```python
from build123d import *

# Parameters (mm, degrees)
SKETCH2_W                           = 10
SKETCH2_H                           = 25
F_5_6_5_6_DIAMETER_HOLE1_AT_2_COUNT = 2
F_5_6_5_6_DIAMETER_HOLE1_AT_2_PITCH = 17.5
F_5_6_5_6_DIAMETER_HOLE1_AT_3_COUNT = 2
F_5_6_5_6_DIAMETER_HOLE1_AT_3_PITCH = 30.310889132
F_5_6_5_6_DIAMETER_HOLE1_AT_4_COUNT = 2
F_5_6_5_6_DIAMETER_HOLE1_AT_4_PITCH = 35
F_5_6_5_6_DIAMETER_HOLE1_AT_5_COUNT = 2
F_5_6_5_6_DIAMETER_HOLE1_AT_5_PITCH = 30.310889132
F_5_6_5_6_DIAMETER_HOLE1_AT_6_COUNT = 2
F_5_6_5_6_DIAMETER_HOLE1_AT_6_PITCH = 17.5
F_0_5MM_CHAMFER1_SIZE               = 0.5


with BuildPart() as part:
    # Sketch2 → Revolve1 (revolve)
    with BuildSketch(Plane.XY, mode=Mode.PRIVATE) as revolve1_sk:
        with Locations((17.5, 12.5)):
            Rectangle(SKETCH2_W, SKETCH2_H)
    revolve1 = revolve(revolve1_sk.sketch.rotate(Axis((0, 0, 0), (0, 1, 0)), 90), axis=Axis((0, 0, 0), (0, 1, 0)))

    # Sketch5 → Ø5.6 (5.6) Diameter Hole1 (revolve, cut)
    with BuildSketch(Plane(origin=(15.155444566, 25, 8.75), x_dir=(0, 0, 1), z_dir=(1, 0, 0))):
        Polygon((0, 0), (0, 9.682409733), (2.8, 8), (2.8, 0), align=None)
    f_5_6_5_6_diameter_hole1 = revolve(axis=Axis((15.155444566, 31.35, 8.75), (0, -1, 0)), mode=Mode.SUBTRACT)

    # Ø5.6 (5.6) Diameter Hole1 at 2: Ø5.6 (5.6) Diameter Hole1 ×2
    with Locations(*[Vector(-0.8660254037844417, 0, 0.49999999999999495) * (i * F_5_6_5_6_DIAMETER_HOLE1_AT_2_PITCH) for i in range(1, F_5_6_5_6_DIAMETER_HOLE1_AT_2_COUNT)]):
        add(f_5_6_5_6_diameter_hole1, mode=Mode.SUBTRACT)

    # Ø5.6 (5.6) Diameter Hole1 at 3: Ø5.6 (5.6) Diameter Hole1 ×2
    with Locations(*[(-i * F_5_6_5_6_DIAMETER_HOLE1_AT_3_PITCH, 0, 0) for i in range(1, F_5_6_5_6_DIAMETER_HOLE1_AT_3_COUNT)]):
        add(f_5_6_5_6_diameter_hole1, mode=Mode.SUBTRACT)

    # Ø5.6 (5.6) Diameter Hole1 at 4: Ø5.6 (5.6) Diameter Hole1 ×2
    with Locations(*[Vector(-0.8660254037844346, 0, -0.5000000000000072) * (i * F_5_6_5_6_DIAMETER_HOLE1_AT_4_PITCH) for i in range(1, F_5_6_5_6_DIAMETER_HOLE1_AT_4_COUNT)]):
        add(f_5_6_5_6_diameter_hole1, mode=Mode.SUBTRACT)

    # Ø5.6 (5.6) Diameter Hole1 at 5: Ø5.6 (5.6) Diameter Hole1 ×2
    with Locations(*[Vector(-0.49999999999999195, 0, -0.8660254037844433) * (i * F_5_6_5_6_DIAMETER_HOLE1_AT_5_PITCH) for i in range(1, F_5_6_5_6_DIAMETER_HOLE1_AT_5_COUNT)]):
        add(f_5_6_5_6_diameter_hole1, mode=Mode.SUBTRACT)

    # Ø5.6 (5.6) Diameter Hole1 at 6: Ø5.6 (5.6) Diameter Hole1 ×2
    with Locations(*[(0, 0, -i * F_5_6_5_6_DIAMETER_HOLE1_AT_6_PITCH) for i in range(1, F_5_6_5_6_DIAMETER_HOLE1_AT_6_COUNT)]):
        add(f_5_6_5_6_diameter_hole1, mode=Mode.SUBTRACT)

    # Mirror1: Revolve1, Ø5.6 (5.6) Diameter Hole1 across plane
    add(revolve1.mirror(Plane.ZX))
    add(f_5_6_5_6_diameter_hole1.mirror(Plane.ZX), mode=Mode.SUBTRACT)

    # Mirror1 copy 1 sketch → Mirror1 copy 1 (revolve, cut)
    with BuildSketch(Plane(origin=(0, -25, 17.5), x_dir=(0, 0, 1), z_dir=(1, 0, 0))):
        Polygon((0, 0), (0, -9.682409733), (2.8, -8), (2.8, 0), align=None)
    revolve(axis=Axis((0, -31.35, 17.5), (0, -1, 0)), mode=Mode.SUBTRACT)

    # Mirror1 copy 2 sketch → Mirror1 copy 2 (revolve, cut)
    with BuildSketch(Plane(origin=(-15.155444566, -25, 8.75), x_dir=(0, 0, 1), z_dir=(1, 0, 0))):
        Polygon((0, 0), (0, -9.682409733), (2.8, -8), (2.8, 0), align=None)
    revolve(axis=Axis((-15.155444566, -31.35, 8.75), (0, -1, 0)), mode=Mode.SUBTRACT)

    # Mirror1 copy 3 sketch → Mirror1 copy 3 (revolve, cut)
    with BuildSketch(Plane(origin=(-15.155444566, -25, -8.75), x_dir=(0, 0, 1), z_dir=(1, 0, 0))):
        Polygon((0, 0), (0, -9.682409733), (2.8, -8), (2.8, 0), align=None)
    revolve(axis=Axis((-15.155444566, -31.35, -8.75), (0, -1, 0)), mode=Mode.SUBTRACT)

    # Mirror1 copy 4 sketch → Mirror1 copy 4 (revolve, cut)
    with BuildSketch(Plane(origin=(0, -25, -17.5), x_dir=(0, 0, 1), z_dir=(1, 0, 0))):
        Polygon((0, 0), (0, -9.682409733), (2.8, -8), (2.8, 0), align=None)
    revolve(axis=Axis((0, -31.35, -17.5), (0, -1, 0)), mode=Mode.SUBTRACT)

    # Mirror1 copy 5 sketch → Mirror1 copy 5 (revolve, cut)
    with BuildSketch(Plane(origin=(15.155444566, -25, -8.75), x_dir=(0, 0, 1), z_dir=(1, 0, 0))):
        Polygon((0, 0), (0, -9.682409733), (2.8, -8), (2.8, 0), align=None)
    revolve(axis=Axis((15.155444566, -31.35, -8.75), (0, -1, 0)), mode=Mode.SUBTRACT)

    # 0,5mm Chamfer1
    f_0_5mm_chamfer1_edges = [part.edges().sort_by_distance(p)[0] for p in [
        (0, -25, 12.5),
        (0, -25, 22.5),
        (0, 25, 22.5),
        (0, 25, 12.5),
    ]]
    chamfer(f_0_5mm_chamfer1_edges, length=F_0_5MM_CHAMFER1_SIZE)


solid = part.part
```
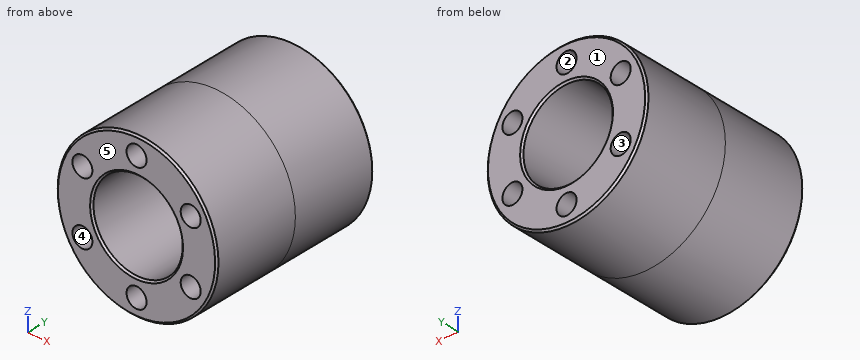
Geometry check sheet. Reference: the model listing, model coordinates, mm. Face numbers are marked on the shaded views. A direction names the side the tool comes from. Round coordinates to 2 decimals unless told otherwise and drop trailing zeros. Order: outer loops, then holes, each group sorted by start corner. A loop starts at its lowest first (then second) coordinate and runs counter-clockwise, first axis right, second up. Notation, with made-up numbers: (-10, 23.5) -> (33, 23.5) arc R25 cw to (33, 56.5) -> close; hole circle Ø6 at (84, 36.25). An arc over 180 degrees is marked (long way). Return JSON: item names as keys, results as strings. Group by question number.
Q1. Tool access check on the marked faces 3, 4 and 5. Record the directions out of +Z, -Z, +X, -X, +Y, -Y that give a thin tool (end or side, any length) a straight path to the whole face; none if there is none.
Q2. Gauge pin test, flat ends, axial feed: pin 1 (8 mm diameter, centred on y = -10, z = -12, fed in from +X); pin 2 (5 mm diameter, centred on x = 15.16, z = 8.75, fed in from -Y); pin 3 (3.5 mm diameter, centred on x = 0, z = 17.5, fed in from -Y); pin 4 (22.5 mm diameter, centred on x = 0, z = 0, fed in from -Y). Record the tip position at first contact, or that the pin passes through.
Q3. Section check B-B, the plane y = 8.5. Record the boundary of the cut face in (x, z).
Q4. Section check A-A, the plane z = 0. Record the boundary of the cut face in (x, y), plus the area to 3 significant figures.
Q5. Material ranges on probe 1 along X at (y, z) = (-21.25, 8.75); probe 2 along X at (y, z) = (11, 0); probe 3 along Z at (x, y) = (-2.5, -20), recorded low to high. Write a range as from..to.
Q6. Release check for a two-part mould opening along Z. For the marked faces 1 and 2 record: released by +Z, released by -Z, zero draft, split by the parting line, or undercut.
Numbers:
{
 "1": {"face 3": "+Y", "face 4": "-Y", "face 5": "+Z, -Z, +X, -X, -Y"},
 "2": {"pin 1": "x = 21.03", "pin 2": "y = -16.82", "pin 3": "y = -16.37", "pin 4": "through"},
 "3": {"outline": "circle Ø45 at (0, 0); hole circle Ø25 at (0, 0)"},
 "4": {"outline": "(-22.5, -24.5) -> (-22, -25) -> (-13, -25) -> (-12.5, -24.5) -> (-12.5, 24.5) -> (-13, 25) -> (-22, 25) -> (-22.5, 24.5) -> close; (12.5, -24.5) -> (13, -25) -> (22, -25) -> (22.5, -24.5) -> (22.5, 24.5) -> (22, 25) -> (13, 25) -> (12.5, 24.5) -> close", "area": "999 mm^2"},
 "5": {"probe 1": "-20.73..-17.96, -12.36..-8.93, 8.93..12.36, 17.96..20.73", "probe 2": "-22.5..-12.5, 12.5..22.5", "probe 3": "-22.36..-18.76, -16.24..-12.25, 12.25..16.24, 18.76..22.36"},
 "6": {"face 1": "zero draft", "face 2": "undercut"}
}
